from build123d import *

# Parameters (mm, degrees)
SKIZZE1_R                       = 27
SKIZZE1_R_2                     = 19
AUFSATZ_LINEAR_AUSTRAGEN1_DEPTH = 79
FASE1_SIZE                      = 0.5


with BuildPart() as part:
    # Skizze1 → Aufsatz-Linear austragen1 (new, symmetric)
    with BuildSketch(Plane.XY):
        Circle(SKIZZE1_R)
        Circle(SKIZZE1_R_2, mode=Mode.SUBTRACT)
    extrude(amount=AUFSATZ_LINEAR_AUSTRAGEN1_DEPTH, both=True)

    # Fase1
    fase1_edges = [part.edges().sort_by_distance(p)[0] for p in [
        (-27, 0, -79),
        (-27, 0, 79),
        (-19, 0, -79),
        (-19, 0, 79),
    ]]
    chamfer(fase1_edges, length=FASE1_SIZE)


solid = part.part
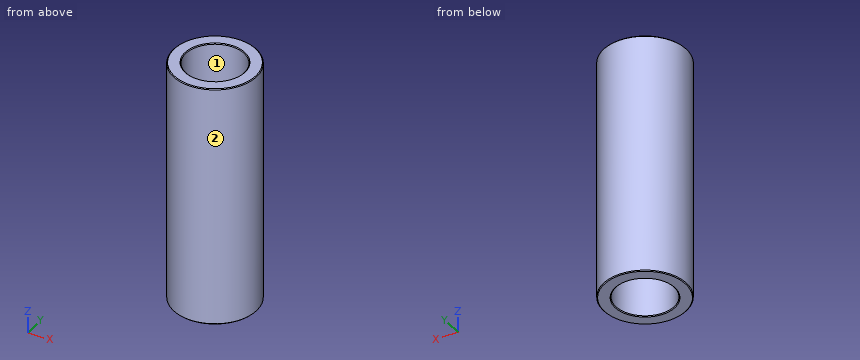
Can you work these out from the model? Positions are in its coordinate system, mm. Face numbers are marked on the shaded views. Give positions to 0.01 mm unless a question says otherwise; leave off trailing zeros. Loops run counter-clockwise (first coordinate to the right, second up) from the corner with the lowest first, then second, coordinate; pieces in that order, holes last. Notation, with made-up numbers: M 46,-25 L 78,-25 A21 cw 78,-1 Z; hole C -13.5,79.25 d5. An arc over 180 degrees is marked long. One line per item, written item: value. Start each with the question number.
1) I'm going to push flat-ended pins straight in: pin 1 (1.5 mm diameter, centred on x = 15, z = -50.5, fed in from -Y); pin 2 (5 mm diameter, centred on y = 5.5, z = 30, fed in from -X); pin 3 (5 mm diameter, centred on y = -17.5, z = 54.5, fed in from +X). Where does each tip first touch, or does it pass through?
2) Thinking about a two-plate mould opening in X: for the marked faces 1 and 2, which applies, +X half, -X half, draft (parallel to the pull), parting line (faces both ways), or undercut?
3) If we section it at A-A, the plane x = 0: Write out the boundary of the cut face in (y, z).
4) If I drill on line 1 (Y direction, x = 0, z = -32.5); line 2 (X direction, y = -1, z = 17.5); line 3 (Y direction, x = 2, z = 66), over which ranges is the centre line in solid material (lowest first)? Write a range as [from, to].
5) If we section it at C-C, the plane z = -3: Write out the boundary of the cut face in (x, y).
Completed:
1. pin 1: stops at y = -22.93
1. pin 2: stops at x = -26.83
1. pin 3: stops at x = 22.45
2. face 1: undercut
2. face 2: parting line
3. outline: M -27,-78.5 L -26.5,-79 L -19.5,-79 L -19,-78.5 L -19,78.5 L -19.5,79 L -26.5,79 L -27,78.5 Z; M 19,-78.5 L 19.5,-79 L 26.5,-79 L 27,-78.5 L 27,78.5 L 26.5,79 L 19.5,79 L 19,78.5 Z
4. line 1: y = [-27, -19], [19, 27]
4. line 2: x = [-26.98, -18.97], [18.97, 26.98]
4. line 3: y = [-26.93, -18.89], [18.89, 26.93]
5. outline: C 0,0 d54; hole C 0,0 d38
